Input: dimensioned drawing with shaded views. Units: mm. Origin: part minimum x, y, z. A direction names the side the tool comes from. Give positions to 0.01 mm unless a question says otherwise; leave off trailing zeros. Write each loop counter-clockwise with the first axis right and the second up, starting at its lowest first coordinate (ties: lowest second). Pieces come first, ordered by that corner, then holes. Notation, with made-up numbers: (21, 41.25) - (29, 41.25) arc R25 cw to (29, 63.25) - close; hole circle Ø8 at (59, 81). An arc over 180 degrees is marked (long way). Answer as CSV lines item,"result".
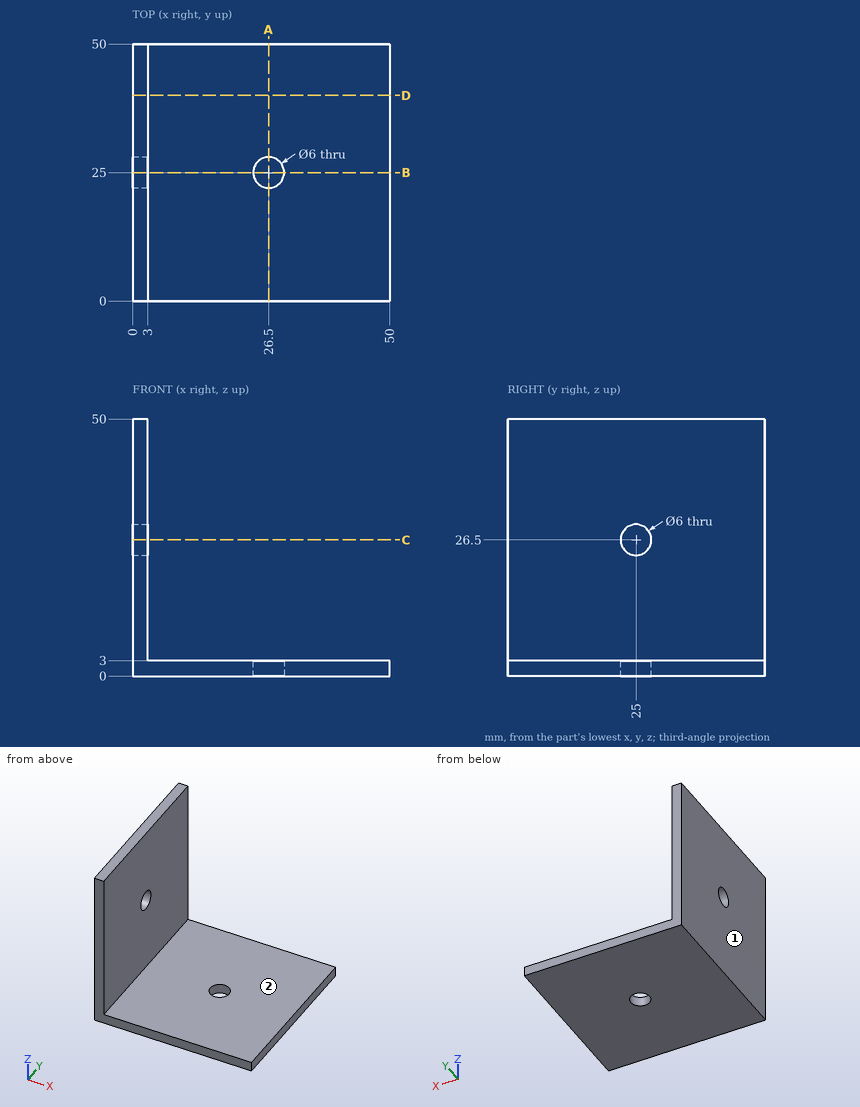
Item 1: Ray query, line 1 (Z direction, x = 2.15, y = 25); line 2 (Y direction, x = 26.5, z = 1.05); line 3 (Z direction, x = 37, y = 27.5). Return the intervals inside material, ascending. Write a range as from..to.
The answers:
line 1,"0..23.5, 29.5..50"
line 2,"0..22, 28..50"
line 3,"0..3"
Item 2: Cut plane C-C on z = 26.5. Return the cut outline in (x, y).
The answers:
outline,"(0, 0) - (3, 0) - (3, 22) - (0, 22) - close; (0, 28) - (3, 28) - (3, 50) - (0, 50) - close"
Item 3: Reachability of the marked faces 1 and 2 from +Z, -Z, +X, -X, +Y, -Y: full face, straight path, thin tool, end or side. Return the list, or none.
The answers:
face 1,"+Z, -Z, -X, +Y, -Y"
face 2,"+Z, +X, +Y, -Y"
Item 4: Cut plane B-B on y = 25. Return the cut outline in (x, z).
The answers:
outline,"(0, 0) - (23.5, 0) - (23.5, 3) - (3, 3) - (3, 23.5) - (0, 23.5) - close; (0, 29.5) - (3, 29.5) - (3, 50) - (0, 50) - close; (29.5, 0) - (50, 0) - (50, 3) - (29.5, 3) - close"
Item 5: Cut plane A-A on x = 26.5. Return the cut outline in (y, z), plus the area to 3 significant figures.
The answers:
outline,"(0, 0) - (22, 0) - (22, 3) - (0, 3) - close; (28, 0) - (50, 0) - (50, 3) - (28, 3) - close"
area,"132 mm²"
Item 6: Cut plane D-D on y = 40. Return the cut outline in (x, z).
The answers:
outline,"(0, 0) - (50, 0) - (50, 3) - (3, 3) - (3, 50) - (0, 50) - close"
Item 7: Contact query for flat-ended pins moving along their axis: pin 1 (1.5 mm diameter, centred on x = 38, y = 5.5, fed in from +Z); pin 2 (5 mm diameter, centred on y = 13, z = 11, fed in from +X). Output: stop coordinate, or through.
The answers:
pin 1,"z = 3"
pin 2,"x = 3"
